Design review of the part shown in the three views and the two pictorial views. Dimensions are in mm from the part's minimum x, y and z. A direction names the side the tool comes from. Give positions to 0.01 mm unless a question says otherwise; leave off trailing zeros. Loops run counter-clockwise (first coordinate to the right, second up) from the corner with the lowest first, then second, coordinate; pieces in that order, holes last. Notation, with made-up numbers: (61, 89.25) - (78, 89.25) arc R35 ccw to (78, 128.25) - close; hole circle Ø4 at (15, 80.25). An arc over 180 degrees is marked (long way). Return JSON: item names as keys, results as strings. Group by question number.
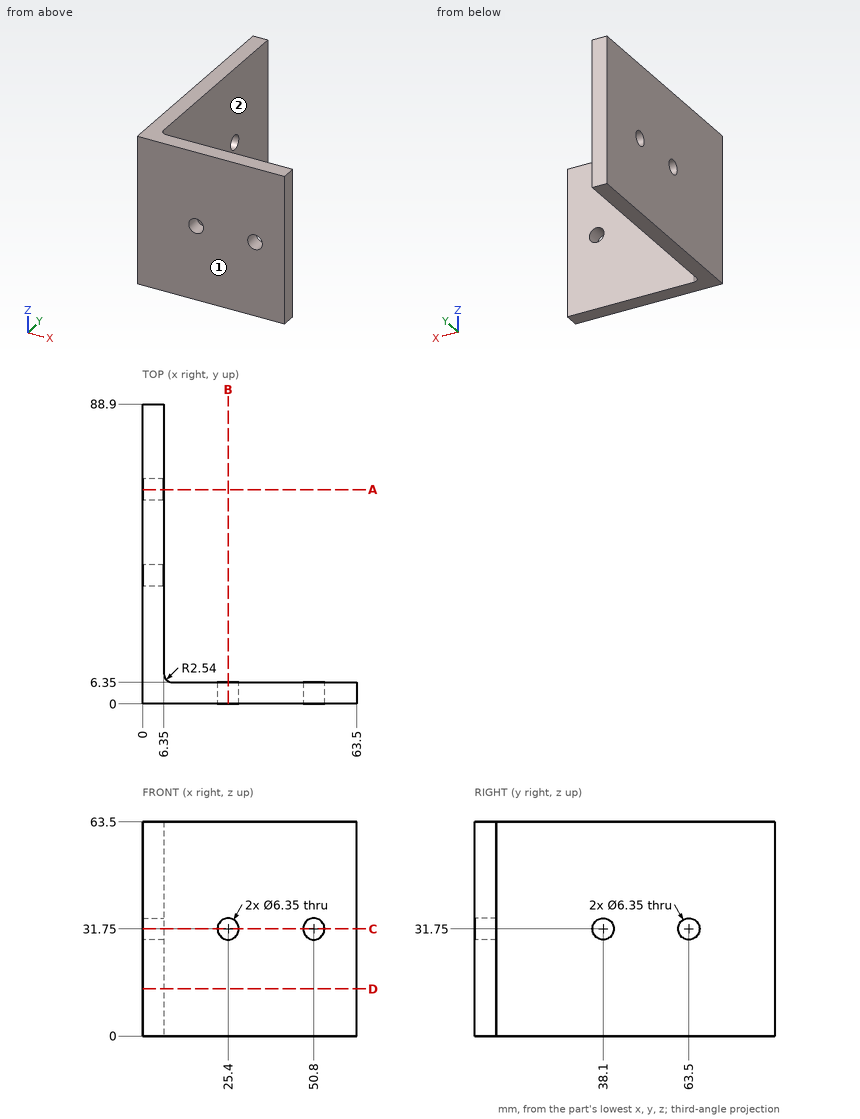
Item 1: Take a section at A-A (y = 63.5). State the section outline as (x, z) points (3 decimals), then the cut area to 3 significant figures.
Item 2: For P1, Ø10, axis at y = 52.5, z = 27.5, coming from the +X side; P2, Ø10, axis at x = 35, z = 8, coming from the +Y side, all flat-tipped, find the tip position at first contact; note any pin that passes through.
Item 3: Take a section at C-C (z = 31.75). State the section outline as (x, y) points (3 decimals), then the cut area to 3 significant figures.
Item 4: Tool access review of the marked faces 1 and 2: name each direction out of +Z, -Z, +X, -X, +Y, -Y from which nothing blocks a thin tool from reaching the whole face with its end or side.
Item 5: For L1, parallel to Y at x = 1.5, z = 31.75 (3 decimals); L2, parallel to Y at x = 18, z = 48; L3, parallel to Z at x = 25.4, y = 5 (3 decimals), list the stretches that pass through material, from the lowest coordinate up. Write a range as from..to.
Item 6: Take a section at D-D (z = 14). State the section outline as (x, y) points, then the cut area to 3 significant figures.
Check sheet entries:
{
 "1": {"outline": "(0, 0) - (6.35, 0) - (6.35, 28.575) - (0, 28.575) - close; (0, 34.925) - (6.35, 34.925) - (6.35, 63.5) - (0, 63.5) - close", "area": "363 mm^2"},
 "2": {"P1": "stops at x = 6.35", "P2": "stops at y = 6.35"},
 "3": {"outline": "(0, 0) - (22.225, 0) - (22.225, 6.35) - (8.89, 6.35) arc R2.54 cw to (6.35, 8.89) - (6.35, 34.925) - (0, 34.925) - close; (0, 41.275) - (6.35, 41.275) - (6.35, 60.325) - (0, 60.325) - close; (0, 66.675) - (6.35, 66.675) - (6.35, 88.9) - (0, 88.9) - close; (28.575, 0) - (47.625, 0) - (47.625, 6.35) - (28.575, 6.35) - close; (53.975, 0) - (63.5, 0) - (63.5, 6.35) - (53.975, 6.35) - close", "area": "768 mm^2"},
 "4": {"face 1": "+Z, -Z, +X, -X, -Y", "face 2": "+Z, -Z, +X, +Y"},
 "5": {"L1": "y = 0..34.925, 41.275..60.325, 66.675..88.9", "L2": "y = 0..6.35", "L3": "z = 0..28.575, 34.925..63.5"},
 "6": {"outline": "(0, 0) - (63.5, 0) - (63.5, 6.35) - (8.89, 6.35) arc R2.54 cw to (6.35, 8.89) - (6.35, 88.9) - (0, 88.9) - close", "area": "929 mm^2"}
}
